Input: part model. Units: mm. Frame: model coordinates. A direction names the side the tool comes from. Round coordinates to 2 decimals unless told otherwise and drop trailing zeros. Use one line per item in the form item = value. Start each with the question number.
Q1. Mould query, pull axis X, two halves, no side actions, for faces 1 (the cylindrical face through (-6.94, -31.24, 12.32)), 2 (the flat face through (-12.152, -2.583, 9.084)), 3 (the flat face through (-7.14, 9.83, 9.08)). Classes: pulls with the +X half, pulls with the -X half, needs draft (parallel to the pull), parting line crosses it, or undercut.
Q2. Section query A-A, the plane x = 8. State how many separate pieces and enclosed holes the cut face has, and give its area (3 significant figures).
Q3. Ray query, line 1 along X through (y, z) = (8.5, 16.25); line 2 along X through (y, z) = (-11, 1.75); line 3 along Y through (x, z) = (-20, 16.5). Return the intervals inside material, ascending.
Q4. First-contact query: P1, Ø2, axis at y = -4.5, z = 9.5, coming from the -X side; P2, Ø5, axis at x = 2.5, z = 5.5, coming from the -Y side; P3, Ø1, axis at y = -7.5, z = 8, coming from the +X side (3 decimals). Flat tips, straight axial feed; report the tip coordinate or a pass-through.
Q5. Access query for faces 4 (the flat face through (11.349, -5.053, 9.084)), 5 (the conical face through (6.421, -2.662, 17.708)). Directions: +Z, -Z, +X, -X, +Y, -Y. A direction counts if a zero-diameter tool reaches every point of the face in a straight line with its end or side. Return the directions, or none.
```python
from build123d import *

# Parameters (mm, degrees)
SKETCH_1_R          = 32
EXTRUDE_1_DEPTH     = 25
SKETCH_2_R          = 25
CUT_EXTRUDE_1_DEPTH = 10
CUT_EXTRUDE_1_TAPER = 68
CUT_EXTRUDE_6_DEPTH = 50


with BuildPart() as part:
    # 스케치1 → 보스-돌출1 (new body)
    with BuildSketch(Plane.XY):
        Circle(SKETCH_1_R)
    extrude(amount=EXTRUDE_1_DEPTH)

    # 스케치2 → 컷-돌출1 (cut)
    with BuildSketch(Plane.XY.offset(25)):
        Circle(SKETCH_2_R)
    extrude(amount=-CUT_EXTRUDE_1_DEPTH, taper=CUT_EXTRUDE_1_TAPER, mode=Mode.SUBTRACT)

    # 스케치4 → 컷-돌출6 (cut)
    with BuildSketch(Plane(origin=(0, 0, 0), x_dir=(-1, 0, 0), z_dir=(0, 0, -1))):
        with BuildLine():
            Line((0, 22), (0, 2.575144905))
            ThreePointArc((0, 2.575144905), (0.666496545, 2.48739897), (1.287572453, 2.230140906))
            Line((1.287572453, 2.230140906), (11, 19.052558883))
            ThreePointArc((11, 19.052558883), (5.694018992, 21.250368178), (0, 22))
        make_face()
        with BuildLine():
            Line((20.098000068, 8.948206148), (2.352511931, 1.047405794))
            ThreePointArc((2.352511931, 1.047405794), (2.001263463, 1.620591199), (1.513632198, 2.083335991))
            Line((1.513632198, 2.083335991), (12.93127555, 17.798373876))
            ThreePointArc((12.93127555, 17.798373876), (17.097211152, 13.845048603), (20.098000068, 8.948206148))
        make_face()
        with BuildLine():
            Line((21.519247216, -4.574057198), (2.51887181, -0.535402731))
            ThreePointArc((2.51887181, -0.535402731), (2.571615758, 0.134772671), (2.449108342, 0.795763539))
            Line((2.449108342, 0.795763539), (20.923243358, 6.798373876))
            ThreePointArc((20.923243358, 6.798373876), (21.969849765, 1.151391037), (21.519247216, -4.574057198))
        make_face()
        with BuildLine():
            Line((14.72087334, -16.349186161), (1.723108272, -1.913705611))
            ThreePointArc((1.723108272, -1.913705611), (2.15969824, -1.402524436), (2.449108342, -0.795763539))
            Line((2.449108342, -0.795763539), (20.923243358, -6.798373876))
            ThreePointArc((20.923243358, -6.798373876), (18.450752495, -11.98205877), (14.72087334, -16.349186161))
        make_face()
        with BuildLine():
            Line((2.299626192, -21.879481698), (0.26917594, -2.561037992))
            ThreePointArc((0.26917594, -2.561037992), (0.922849399, -2.404104879), (1.513632198, -2.083335991))
            Line((1.513632198, -2.083335991), (12.93127555, -17.798373876))
            ThreePointArc((12.93127555, -17.798373876), (7.88409489, -20.538769383), (2.299626192, -21.879481698))
        make_face()
        with BuildLine():
            Line((-11, -19.052558883), (-1.287572453, -2.230140906))
            ThreePointArc((-1.287572453, -2.230140906), (-0.666496545, -2.48739897), (0, -2.575144905))
            Line((0, -2.575144905), (0, -22))
            ThreePointArc((0, -22), (-5.694018992, -21.250368178), (-11, -19.052558883))
        make_face()
        with BuildLine():
            Line((-20.098000068, -8.948206148), (-2.352511931, -1.047405794))
            ThreePointArc((-2.352511931, -1.047405794), (-2.001263463, -1.620591199), (-1.513632198, -2.083335991))
            Line((-1.513632198, -2.083335991), (-12.93127555, -17.798373876))
            ThreePointArc((-12.93127555, -17.798373876), (-17.097211152, -13.845048603), (-20.098000068, -8.948206148))
        make_face()
        with BuildLine():
            Line((-21.519247216, 4.574057198), (-2.51887181, 0.535402731))
            ThreePointArc((-2.51887181, 0.535402731), (-2.571615758, -0.134772671), (-2.449108342, -0.795763539))
            Line((-2.449108342, -0.795763539), (-20.923243358, -6.798373876))
            ThreePointArc((-20.923243358, -6.798373876), (-21.969849765, -1.151391037), (-21.519247216, 4.574057198))
        make_face()
        with BuildLine():
            Line((-14.72087334, 16.349186161), (-1.723108272, 1.913705611))
            ThreePointArc((-1.723108272, 1.913705611), (-2.15969824, 1.402524436), (-2.449108342, 0.795763539))
            Line((-2.449108342, 0.795763539), (-20.923243358, 6.798373876))
            ThreePointArc((-20.923243358, 6.798373876), (-18.450752495, 11.98205877), (-14.72087334, 16.349186161))
        make_face()
        with BuildLine():
            Line((-2.299626192, 21.879481698), (-0.26917594, 2.561037992))
            ThreePointArc((-0.26917594, 2.561037992), (-0.922849399, 2.404104879), (-1.513632198, 2.083335991))
            Line((-1.513632198, 2.083335991), (-12.93127555, 17.798373876))
            ThreePointArc((-12.93127555, 17.798373876), (-7.88409489, 20.538769383), (-2.299626192, 21.879481698))
        make_face()
    extrude(amount=-CUT_EXTRUDE_6_DEPTH, mode=Mode.SUBTRACT)


solid = part.part
```
Results found:
q1.face_1 = parting line crosses it
q1.face_2 = undercut
q1.face_3 = undercut
q2.separate_pieces = 6
q2.enclosed_holes = 0
q2.area = 657 mm²
q3.line_1 = -30.85 to -19.09, -6.18 to -4.91, 0 to 0.89, 6.18 to 7.65, 20.29 to 30.85
q3.line_2 = -30.05 to -19.05, -9.9 to -7.99, -1.16 to 0, 6.35 to 7.99, 19.05 to 30.05
q3.line_3 = -24.98 to -9.17, -6.5 to -4.25, 6.5 to 8.9, 9.17 to 24.98
q4.P1 = -31.81
q4.P2 = -32
q4.P3 = 31.225
q5.face_4 = +Z, -Z
q5.face_5 = +Z
